Here's how the part is built. I have some questions about the finished solid (model axes, mm). Round coordinates to 2 decimals unless told otherwise and drop trailing zeros. Order: outer loops, then holes, each group sorted by start corner. A loop starts at its lowest first (then second) coordinate and runs counter-clockwise, first axis right, second up. Notation, with made-up numbers: (-27.5, -37.75) -> (-19.5, -37.75) arc R17 ccw to (-19.5, -9.75) -> close; hole circle Ø1 at (-36, 30.25). An arc over 180 degrees is marked (long way). One line per item, written item: value.
```python
from build123d import *

# Parameters (mm, degrees)
SKETCH1_R                            = 40
BOSS_EXTRUDE1_DEPTH                  = 60.075
TAP_DRILL_FOR_M6X1_0_TAP1_AT_2_COUNT = 2
TAP_DRILL_FOR_M6X1_0_TAP1_AT_2_PITCH = 30
TAP_DRILL_FOR_M6X1_0_TAP1_AT_3_COUNT = 2
TAP_DRILL_FOR_M6X1_0_TAP1_AT_3_PITCH = 51.961524227
TAP_DRILL_FOR_M6X1_0_TAP1_AT_4_COUNT = 2
TAP_DRILL_FOR_M6X1_0_TAP1_AT_4_PITCH = 60
TAP_DRILL_FOR_M6X1_0_TAP1_AT_5_COUNT = 2
TAP_DRILL_FOR_M6X1_0_TAP1_AT_5_PITCH = 51.961524227
TAP_DRILL_FOR_M6X1_0_TAP1_AT_6_COUNT = 2
TAP_DRILL_FOR_M6X1_0_TAP1_AT_6_PITCH = 30


with BuildPart() as part:
    # Sketch1 → Boss-Extrude1 (new body)
    with BuildSketch(Plane(origin=(0, 0, 0), x_dir=(1, 0, 0), z_dir=(0, 1, 0))):
        with Locations(Location((0, 0, 0), (0, 0, 270))):
            Circle(SKETCH1_R)
    boss_extrude1 = extrude(amount=BOSS_EXTRUDE1_DEPTH)

    # Sketch4 → Tap Drill for M6x1.0 Tap1 (revolve, cut)
    with BuildSketch(Plane(origin=(25.980762114, 0, 15), x_dir=(0, 0, -1), z_dir=(1, 0, 0))):
        Polygon((0, 0), (0, 11.502151548), (2.5, 10), (2.5, 0), align=None)
    tap_drill_for_m6x1_0_tap1 = revolve(axis=Axis((25.980762114, -6.35, 15), (0, 1, 0)), mode=Mode.SUBTRACT)

    # Tap Drill for M6x1.0 Tap1 at 2: Tap Drill for M6x1.0 Tap1 ×2
    with Locations(*[(0, 0, -i * TAP_DRILL_FOR_M6X1_0_TAP1_AT_2_PITCH) for i in range(1, TAP_DRILL_FOR_M6X1_0_TAP1_AT_2_COUNT)]):
        add(tap_drill_for_m6x1_0_tap1, mode=Mode.SUBTRACT)

    # Tap Drill for M6x1.0 Tap1 at 3: Tap Drill for M6x1.0 Tap1 ×2
    with Locations(*[Vector(-0.5000000000000001, 0, -0.8660254037844386) * (i * TAP_DRILL_FOR_M6X1_0_TAP1_AT_3_PITCH) for i in range(1, TAP_DRILL_FOR_M6X1_0_TAP1_AT_3_COUNT)]):
        add(tap_drill_for_m6x1_0_tap1, mode=Mode.SUBTRACT)

    # Tap Drill for M6x1.0 Tap1 at 4: Tap Drill for M6x1.0 Tap1 ×2
    with Locations(*[Vector(-0.8660254037844389, 0, -0.4999999999999995) * (i * TAP_DRILL_FOR_M6X1_0_TAP1_AT_4_PITCH) for i in range(1, TAP_DRILL_FOR_M6X1_0_TAP1_AT_4_COUNT)]):
        add(tap_drill_for_m6x1_0_tap1, mode=Mode.SUBTRACT)

    # Tap Drill for M6x1.0 Tap1 at 5: Tap Drill for M6x1.0 Tap1 ×2
    with Locations(*[(-i * TAP_DRILL_FOR_M6X1_0_TAP1_AT_5_PITCH, 0, 0) for i in range(1, TAP_DRILL_FOR_M6X1_0_TAP1_AT_5_COUNT)]):
        add(tap_drill_for_m6x1_0_tap1, mode=Mode.SUBTRACT)

    # Tap Drill for M6x1.0 Tap1 at 6: Tap Drill for M6x1.0 Tap1 ×2
    with Locations(*[Vector(-0.8660254037844386, 0, 0.5000000000000001) * (i * TAP_DRILL_FOR_M6X1_0_TAP1_AT_6_PITCH) for i in range(1, TAP_DRILL_FOR_M6X1_0_TAP1_AT_6_COUNT)]):
        add(tap_drill_for_m6x1_0_tap1, mode=Mode.SUBTRACT)

    # Mirror1: Boss-Extrude1, Tap Drill for M6x1.0 Tap1 across plane
    add(boss_extrude1.mirror(Plane.ZX.offset(60.075)))
    add(tap_drill_for_m6x1_0_tap1.mirror(Plane.ZX.offset(60.075)), mode=Mode.SUBTRACT)

    # Mirror1 copy 1 sketch → Mirror1 copy 1 (revolve, cut)
    with BuildSketch(Plane(origin=(25.980762114, 120.15, -15), x_dir=(0, 0, -1), z_dir=(1, 0, 0))):
        Polygon((0, 0), (0, -11.502151548), (2.5, -10), (2.5, 0), align=None)
    revolve(axis=Axis((25.980762114, 126.5, -15), (0, 1, 0)), mode=Mode.SUBTRACT)

    # Mirror1 copy 2 sketch → Mirror1 copy 2 (revolve, cut)
    with BuildSketch(Plane(origin=(0, 120.15, -30), x_dir=(0, 0, -1), z_dir=(1, 0, 0))):
        Polygon((0, 0), (0, -11.502151548), (2.5, -10), (2.5, 0), align=None)
    revolve(axis=Axis((0, 126.5, -30), (0, 1, 0)), mode=Mode.SUBTRACT)

    # Mirror1 copy 3 sketch → Mirror1 copy 3 (revolve, cut)
    with BuildSketch(Plane(origin=(-25.980762114, 120.15, -15), x_dir=(0, 0, -1), z_dir=(1, 0, 0))):
        Polygon((0, 0), (0, -11.502151548), (2.5, -10), (2.5, 0), align=None)
    revolve(axis=Axis((-25.980762114, 126.5, -15), (0, 1, 0)), mode=Mode.SUBTRACT)

    # Mirror1 copy 4 sketch → Mirror1 copy 4 (revolve, cut)
    with BuildSketch(Plane(origin=(-25.980762114, 120.15, 15), x_dir=(0, 0, -1), z_dir=(1, 0, 0))):
        Polygon((0, 0), (0, -11.502151548), (2.5, -10), (2.5, 0), align=None)
    revolve(axis=Axis((-25.980762114, 126.5, 15), (0, 1, 0)), mode=Mode.SUBTRACT)

    # Mirror1 copy 5 sketch → Mirror1 copy 5 (revolve, cut)
    with BuildSketch(Plane(origin=(0, 120.15, 30), x_dir=(0, 0, -1), z_dir=(1, 0, 0))):
        Polygon((0, 0), (0, -11.502151548), (2.5, -10), (2.5, 0), align=None)
    revolve(axis=Axis((0, 126.5, 30), (0, 1, 0)), mode=Mode.SUBTRACT)


solid = part.part
```
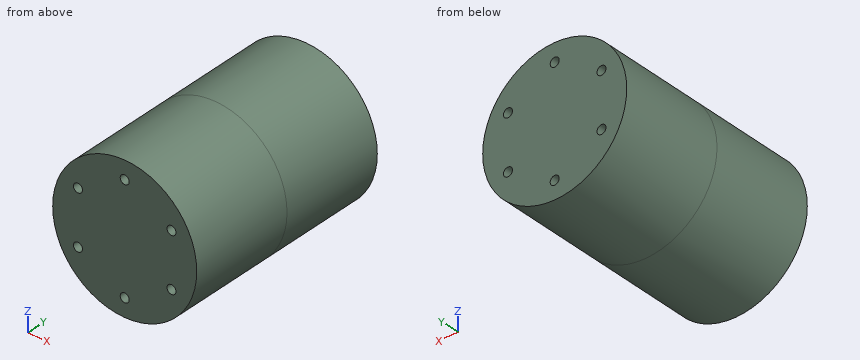
Q1. I want a section at A-A on y = 16.5. Write out the boundary of the cut face in (x, z).
Answers:
outline: circle Ø80 at (0, 0)
Q2. I need wall thicknesses on line 1 along X through (y, z) = (3.5, -15); line 2 along X through (y, z) = (114, -30); line 3 along Z through (x, y) = (28, 111). Which ranges of each line are inside material? Lowest first, please.
Answers:
line 1: -37.08 to -28.48, -23.48 to 23.48, 28.48 to 37.08
line 2: -26.46 to -2.5, 2.5 to 26.46
line 3: -28.57 to -16.47, -13.53 to 13.53, 16.47 to 28.57
Q3. For P1, Ø4.5, axis at x = 25.98, z = -15, coming from the -Y side; P2, Ø3, axis at x = 25.98, z = -15, coming from the +Y side; P3, Ø2, axis at y = 73, z = 11.5, coming from the -X side, each with a flat end and sliding along its axis, tell me the tip position at first contact or that it passes through.
Answers:
P1: y = 10.15
P2: y = 109.55
P3: x = -38.6
Q4. I want a section at C-C on z = 10.5. Write out the boundary of the cut face in (x, y).
Answers:
outline: (-38.6, 0) -> (38.6, 0) -> (38.6, 120.15) -> (-38.6, 120.15) -> close
Q5. I want a section at B-B on x = -30. Write out the boundary of the cut face in (y, z).
Answers:
outline: (0, -26.46) -> (120.15, -26.46) -> (120.15, 26.46) -> (0, 26.46) -> close
